Design review of the part built by this model. Coordinates are the model's own, in mm. Face numbers are marked on the shaded views. A direction names the side the tool comes from. Round coordinates to 2 decimals unless told otherwise and drop trailing zeros. Write each loop counter-clockwise with the first axis right and the second up, starting at its lowest first coordinate (ties: lowest second). Pieces come first, ordered by that corner, then holes. Notation, with made-up numbers: M -27,41.25 L -11,41.25 A32 cw -11,68.25 Z; hole C 67,85.25 d4. An arc over 180 degrees is marked long. One line per question, with ' | ' between items. Start each with the question number.
Item 1: Machinability: for the marked faces 4, 5 and 6, which of the approach directions +Z, -Z, +X, -X, +Y, -Y give a long, thin tool a straight path to every point of the face, cutting with its end or side? Answer none if there is none.
Item 2: Add section C-C, the plane z = 0.8. State the section outline as (x, y) points, and give its area (3 significant figures).
Item 3: For L1, parallel to Y at x = 0.5, z = 0.35; L2, parallel to Z at x = 2.5, y = 0.1; L3, parallel to X at y = -0.5, z = 1.65, list the stretches that pass through material, from the lowest coordinate up.
Item 4: Add section A-A, the plane z = 1.9. State the section outline as (x, y) points.
Item 5: Add section B-B, the plane y = 0. State the section outline as (x, z) points.
Item 6: Insertion check: pin 1 Ø0.8 at (x, z) = (0, 2.5) entering from +Y; pin 2 Ø1.1 at (x, z) = (0, 2) entering from -Y. Each pin has a flat end and moves straight along its axis. Give the tip position at first contact, or say it passes through.
Item 7: Add section D-D, the plane z = 3.2. State the section outline as (x, y) points.
Item 8: Draft analysis for pull direction Y (two halves, no side actions). For the marked faces 1, 2 and 3, state which applies: released by +Y, released by -Y, zero draft, split by the parting line, or undercut.
```python
from build123d import *

# Parameters (mm, degrees)
EXTRUDE_1_DEPTH     = 1.4
EXTRUDE_2_DEPTH     = 2
SKETCH_4_W          = 1.6
SKETCH_4_H          = 1.2
CUT_EXTRUDE_1_DEPTH = 2


with BuildPart() as part:
    # 草图2 → 凸台-拉伸1 (new body)
    with BuildSketch(Plane.XY):
        with BuildLine():
            Line((-2, 1.4), (2, 1.4))
            ThreePointArc((2, 1.4), (3.4, 0), (2, -1.4))
            Line((2, -1.4), (-2, -1.4))
            ThreePointArc((-2, -1.4), (-3.4, 0), (-2, 1.4))
        make_face()
    extrude(amount=EXTRUDE_1_DEPTH)

    # 草图3 → 凸台-拉伸2 (add)
    with BuildSketch(Plane.XY.offset(1.4)):
        with BuildLine():
            Line((-0.5, 0.9), (0.5, 0.9))
            ThreePointArc((0.5, 0.9), (1.4, 0), (0.5, -0.9))
            Line((0.5, -0.9), (-0.5, -0.9))
            ThreePointArc((-0.5, -0.9), (-1.4, 0), (-0.5, 0.9))
        make_face()
    extrude(amount=EXTRUDE_2_DEPTH)

    # 草图4 → 切除-拉伸1 (cut)
    with BuildSketch(Plane(origin=(0, 0, 0), x_dir=(-1, 0, 0), z_dir=(0, 0, -1))):
        Rectangle(SKETCH_4_W, SKETCH_4_H)
    extrude(amount=-CUT_EXTRUDE_1_DEPTH, mode=Mode.SUBTRACT)


solid = part.part
```
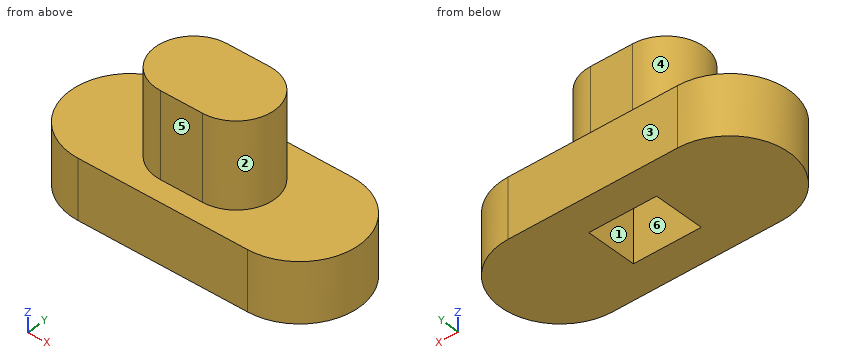
Computed values:
1) face 4: +Z, -X | face 5: +Z, +X, -X, -Y | face 6: -Z
2) outline: M -2,-1.4 L 2,-1.4 A1.4 ccw 2,1.4 L -2,1.4 A1.4 ccw Z; hole M -0.8,-0.6 L 0.8,-0.6 L 0.8,0.6 L -0.8,0.6 Z | area: 15.4 mm^2
3) L1: y = -1.4 to -0.6, 0.6 to 1.4 | L2: z = 0 to 1.4 | L3: x = -1.25 to -0.8, 0.8 to 1.25
4) outline: M -0.5,-0.9 L 0.5,-0.9 A0.9 ccw 0.5,0.9 L -0.5,0.9 A0.9 ccw Z; hole M -0.8,-0.6 L 0.8,-0.6 L 0.8,0.6 L -0.8,0.6 Z
5) outline: M -3.4,0 L -0.8,0 L -0.8,2 L 0.8,2 L 0.8,0 L 3.4,0 L 3.4,1.4 L 1.4,1.4 L 1.4,3.4 L -1.4,3.4 L -1.4,1.4 L -3.4,1.4 Z
6) pin 1: stops at y = 0.9 | pin 2: stops at y = -0.9
7) outline: M -0.5,-0.9 L 0.5,-0.9 A0.9 ccw 0.5,0.9 L -0.5,0.9 A0.9 ccw Z
8) face 1: undercut | face 2: split by the parting line | face 3: released by +Y
